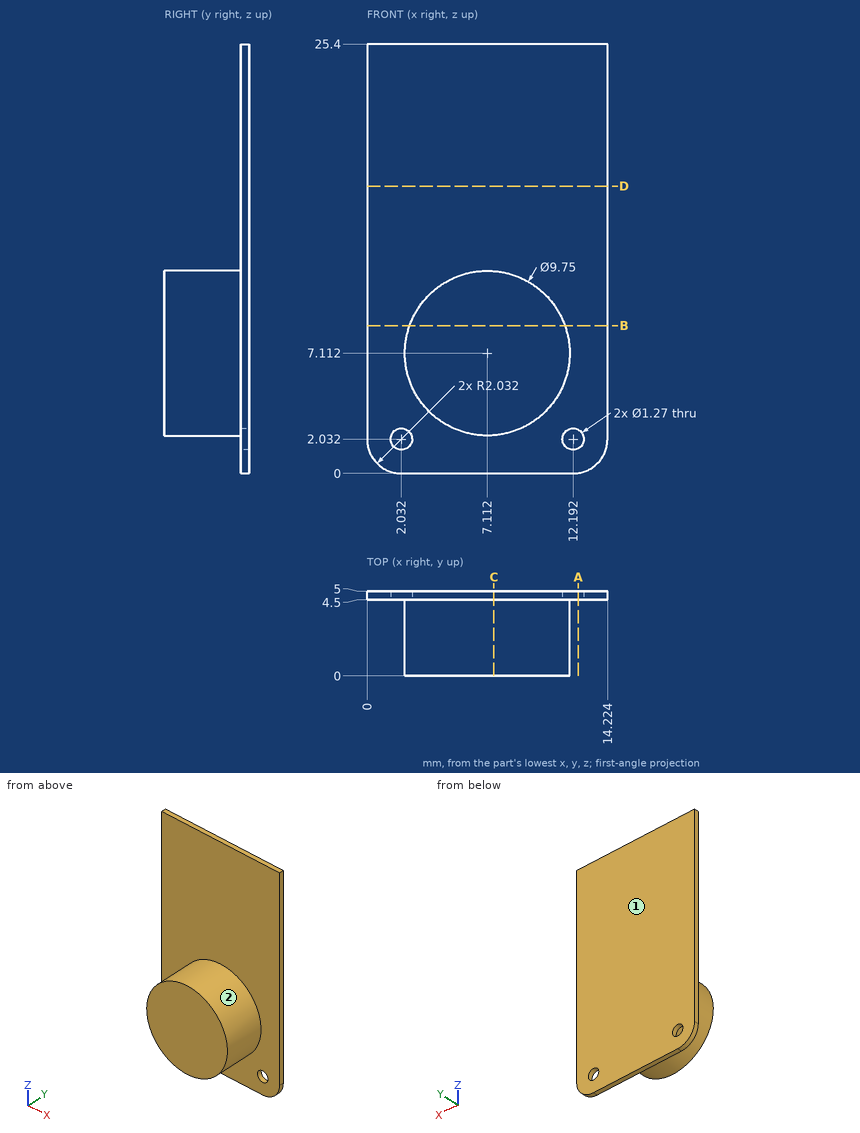
Study the drawing (mm; zero at the part's minimum x, y, z) and answer. A direction names the side the tool comes from. Coordinates: 2 decimals unless noted, no trailing zeros. Loops run counter-clockwise (first coordinate to the right, second up) from the corner with the lowest first, then second, coordinate; pieces in that order, holes last. Notation, with made-up numbers: (23, 41.5) -> (61, 41.5) arc R29 ccw to (61, 75.5) -> close; hole circle Ø3 at (-26, 72). An arc over 180 degrees is marked (long way). Answer in a Markdown table with one row per item. Add a question column.
1. Flat-ended cylindrical pins translate along their axes: P1, Ø2, axis at x = 12, y = 2.5, coming from the -Z side; P2, Ø4.5, axis at x = 8, z = 18.5, coming from the -Y side. Find the tip coordinate at first contact, or state that the pin passes through.
2. Consider line 1 (Y direction, x = 9, z = 17); line 2 (Z direction, x = 9, y = 2.05); line 3 (Z direction, x = 11, y = 2.45). Determine where each line is inside the solid, lowest interval first. Write a range as [from, to].
3. The part is cut by section C-C, the plane x = 7.5. Write down the section's boundary in (y, z), then the cut area to 3 significant figures.
4. The part is cut by section A-A, the plane x = 12.5. Write down the section's boundary in (y, z).
5. The part is cut by section B-B, the plane z = 8.75. Write down the section's boundary in (x, y).
6. For the marked faces 1 and 2, determine the directions among +Z, -Z, +X, -X, +Y, -Y from which every point of the face is accessible in a straight line to the end or side of a thin tool.
7. The part is cut by section D-D, the plane z = 17. Write down the section's boundary in (x, y), then the cut area to 3 significant figures.
Answer below:
| question | item | result |
|---|---|---|
| 1 | P1 | z = 4.17 |
| 1 | P2 | y = 4.5 |
| 2 | line 1 | [4.5, 5] |
| 2 | line 2 | [2.62, 11.61] |
| 2 | line 3 | [4.17, 10.05] |
| 3 | outline | (0, 2.25) -> (4.5, 2.25) -> (4.5, 0) -> (5, 0) -> (5, 25.4) -> (4.5, 25.4) -> (4.5, 11.97) -> (0, 11.97) -> close |
| 3 | area | 56.4 mm2 |
| 4 | outline | (4.5, 0.02) -> (5, 0.02) -> (5, 1.48) -> (4.5, 1.48) -> close; (4.5, 2.59) -> (5, 2.59) -> (5, 25.4) -> (4.5, 25.4) -> close |
| 5 | outline | (0, 4.5) -> (2.52, 4.5) -> (2.52, 0) -> (11.7, 0) -> (11.7, 4.5) -> (14.22, 4.5) -> (14.22, 5) -> (0, 5) -> close |
| 6 | face 1 | +Z, -Z, +X, -X, +Y |
| 6 | face 2 | -Y |
| 7 | outline | (0, 4.5) -> (14.22, 4.5) -> (14.22, 5) -> (0, 5) -> close |
| 7 | area | 7.11 mm2 |
